Geometry: final body of the model. Coordinates: model frame, mm. A direction names the side the tool comes from. Give positions to 0.01 mm unless a question says otherwise; leave off trailing zeros. Loops run counter-clockwise (first coordinate to the right, second up) from the corner with the lowest first, then second, coordinate; pieces in that order, holes last. Notation, with made-up numbers: (25.5, 71.25) -> (61.5, 71.25) arc R27 cw to (61.5, 103.25) -> close; hole circle Ø4 at (77, 68.5). An arc over 180 degrees is marked (long way). One line per item, written item: value. Start each with the question number.
from build123d import *

# Parameters (mm, degrees)
ESQUISSE2_R             = 3.25
ENL_V_MAT_EXTRU_1_DEPTH = 10.5
ENL_V_START             = -2.5
ESQUISSE3_R             = 5.25
ENL_V_MAT_EXTRU_2_DEPTH = 7.880262221


with BuildPart() as part:
    # Esquisse1 → Révolution1 (revolve)
    with BuildSketch(Plane.XY, mode=Mode.PRIVATE) as r_volution1_sk:
        with BuildLine():
            Line((-16, 6.5), (-16, 5.5))
            Line((-16, 5.5), (-14.25, 5.5))
            Line((-14.25, 5.5), (-14.25, 4.5))
            ThreePointArc((-14.25, 4.5), (-9.106739847, 3.315312536), (-5, 0))
            Line((-5, 0), (0, 0))
            Line((0, 0), (0, 9.5))
            ThreePointArc((0, 9.5), (-8.139410298, 8.74352159), (-16, 6.5))
        make_face()
    revolve(r_volution1_sk.sketch.rotate(Axis((0, 18.461307074, 0), (0, -1, 0)), 270), axis=Axis((0, 18.461307074, 0), (0, -1, 0)))  # turned: the seam where the file's is

    # Esquisse2 → Enlèv. mat.-Extru.1 (cut, through all)
    with BuildSketch(Plane.XZ):
        with Locations(Location((0, 0, 0), (0, 0, 270))):  # turned: the seam where the file's is
            Circle(ESQUISSE2_R)
    extrude(amount=-ENL_V_MAT_EXTRU_1_DEPTH, mode=Mode.SUBTRACT)

    # Esquisse3 → Enlèv. mat.-Extru.2 (cut, through all)
    with BuildSketch(Plane.XZ.offset(ENL_V_START)):
        with Locations(Location((0, 0, 0), (0, 0, 270))):  # turned: the seam where the file's is
            Circle(ESQUISSE3_R)
    extrude(amount=-ENL_V_MAT_EXTRU_2_DEPTH, mode=Mode.SUBTRACT)


solid = part.part
Item 1: Section C-C, the plane y = 3.25. Output: boundary loops of the cut face in (x, z), then the cut area to 3 significant figures.
Item 2: Section A-A, the plane x = 0. Output: boundary loops of the cut face in (y, z), then the cut area to 3 significant figures.
Item 3: Mould query, pull axis X, two halves, no side actions, for faces 1 (the face through (1, 0, 3.3)), 2 (the face through (1.6, 5.8, -5)), 3 (the face through (13.91, 4.99, -3.09)). Classes: pulls with the +X half, pulls with the -X half, needs draft (parallel to the pull), parting line crosses it, or undercut.
Item 4: Section B-B, the plane z = 0. Output: boundary loops of the cut face in (x, y), then the cut area to 3 significant figures.
Item 5: Section D-D, the plane y = 7. Output: boundary loops of the cut face in (x, z), then the cut area to 3 significant figures.
Item 6: Access query for faces 4 (the face through (-3.4, 2.5, 0.1)), 5 (the face through (11, 5.5, -10)), 6 (the face through (15.62, 5.99, -3.47)). Directions: +Z, -Z, +X, -X, +Y, -Y. A direction counts if a zero-diameter tool reaches every point of the face in a straight line with its end or side. Return the directions, or none.
Item 7: Ray query, line 1 along Z through (x, y) = (2.5, 3.25); line 2 along X through (y, z) = (3.5, -2); line 3 along X through (y, z) = (1.95, 0). Return the intervals inside material, ascending. Write a range as [from, to].
Item 8: Pin query (flat end, axial travel): pin 1 (1.5 mm diameter, centred on x = -11.5, z = -1.5, fed in from +Y); pin 2 (5 mm diameter, centred on x = 0.5, z = 2.5, fed in from +Y); pin 3 (6 mm diameter, centred on x = 9, z = 7, fed in from -Y). Return the tip coordinate at first contact, or that it passes through.
Geometry check:
1. outline: circle Ø17.95 at (0, 0); hole circle Ø10.5 at (0, 0)
1. area: 166 mm2
2. outline: (0, -5) arc R11.76 cw to (4.5, -14.25) -> (5.5, -14.25) -> (5.5, -16) -> (6.5, -16) arc R44.17 ccw to (9.19, -5.25) -> (2.5, -5.25) -> (2.5, -3.25) -> (0, -3.25) -> close; (0, 3.25) -> (2.5, 3.25) -> (2.5, 5.25) -> (9.19, 5.25) arc R44.17 ccw to (6.5, 16) -> (5.5, 16) -> (5.5, 14.25) -> (4.5, 14.25) arc R11.76 cw to (0, 5) -> close
2. area: 106 mm2
3. face 1: needs draft
3. face 2: undercut
3. face 3: parting line crosses it
4. outline: (-16, 5.5) -> (-14.25, 5.5) -> (-14.25, 4.5) arc R11.76 cw to (-5, 0) -> (-3.25, 0) -> (-3.25, 2.5) -> (-5.25, 2.5) -> (-5.25, 9.19) arc R44.17 ccw to (-16, 6.5) -> close; (3.25, 0) -> (5, 0) arc R11.76 cw to (14.25, 4.5) -> (14.25, 5.5) -> (16, 5.5) -> (16, 6.5) arc R44.17 ccw to (5.25, 9.19) -> (5.25, 2.5) -> (3.25, 2.5) -> close
4. area: 106 mm2
5. outline: circle Ø29.3 at (0, 0); hole circle Ø10.5 at (0, 0)
5. area: 588 mm2
6. face 4: +Y
6. face 5: -Y
6. face 6: +Y, -Y
7. line 1: z = [-8.62, -4.62], [4.62, 8.62]
7. line 2: x = [-9.29, -4.85], [4.85, 9.29]
7. line 3: x = [-6.94, -3.25], [3.25, 6.94]
8. pin 1: stops at y = 8.15
8. pin 2: stops at y = 2.5
8. pin 3: stops at y = 2.94
